The listing builds one solid part. Answer for the finished solid, in the listing's coordinates (mm). Face numbers are marked on the shaded views. Give positions to 0.01 mm unless a question says otherwise; leave off trailing zeros. Loops run counter-clockwise (first coordinate to the right, second up) from the corner with the lowest first, then second, coordinate; pieces in that order, holes last. Notation, with made-up numbers: (34, -39) - (49, -39) arc R24 ccw to (49, -28) - close; hole circle Ø8 at (84.5, -18). An arc over 180 degrees is marked (long way). Answer as CSV lines item,"result". Start each with the question number.
1) For a pull along Y with two mould halves and no side action, classify the marked faces 1, 2, 3 and 4 as pulls with the +Y half, pulls with the -Y half, needs draft (parallel to the pull), parting line crosses it, or undercut.
2) Find the intervals of material crossed by line 1 along Y through (x, z) = (2.3, 18); line 2 along X through (y, z) = (4, -6.5); line 3 along X through (y, z) = (13.5, -3.5), in increasing order.
3) Flat-ended cylindrical pins translate along their axes: pin 1 (2 mm diameter, centred on y = 14.5, z = -0.5, fed in from +X); pin 2 (1.5 mm diameter, centred on x = 1.5, y = -4.5, fed in from +Z); pin 3 (3 mm diameter, centred on y = -8.5, z = -1, fed in from -X). Find the tip coordinate at first contact, or state that the pin passes through.
4) A cutting plane is placed at B-B (z = 7). Determine the outline of the cut face in (x, y).
5) A cutting plane is placed at A-A (y = 0). Determine the outline of the cut face in (x, z).
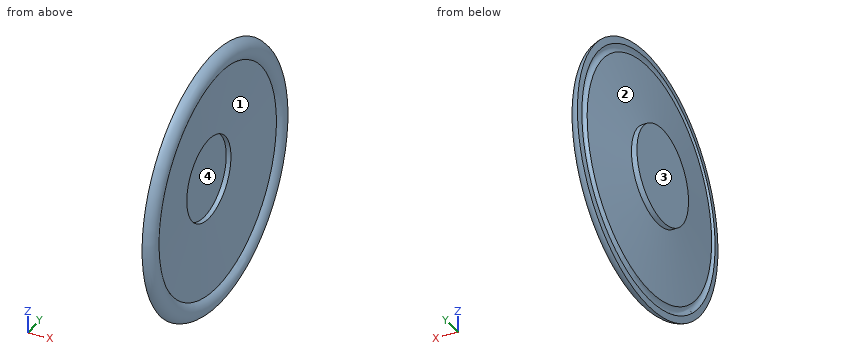
```python
from build123d import *


with BuildPart() as part:
    # Sketch1 → Revolve-Thin3 (revolve)
    with BuildSketch(Plane(origin=(0, 0, 0), x_dir=(1, 0, 0), z_dir=(0, 1, 0))):
        with BuildLine():
            Line((-0.794424497, -7), (-0.794424497, 0))
            Line((-0.794424497, 0), (0, 0))
            Line((0, 0), (1.142372775, 9.900564049))
            ThreePointArc((1.142372775, 9.900564049), (1.801141725, 10.423035974), (1.278669799, 11.081804924))
            Line((1.278669799, 11.081804924), (1.393293907, 12.07521386))
            ThreePointArc((1.393293907, 12.07521386), (2.765201716, 10.845477658), (2.061567501, 9.142750125))
            Line((2.061567501, 9.142750125), (0.891250179, -1))
            Line((0.891250179, -1), (0.205575503, -1))
            Line((0.205575503, -1), (0.205575503, -7))
            Line((0.205575503, -7), (-0.794424497, -7))
        make_face()
    revolve(axis=Axis((-0.794424497, 0, 7), (1, 0, 0)))


solid = part.part
```
Ans:
1,face 1,"undercut"
1,face 2,"parting line crosses it"
1,face 3,"needs draft"
1,face 4,"undercut"
2,line 1,"-15.07 to -12.07, 12.07 to 15.07"
2,line 2,"0.82 to 1.82"
2,line 3,"1.66 to 2.76"
3,pin 1,"x = 2.8"
3,pin 2,"z = 25.7"
3,pin 3,"x = 0.37"
4,outline,"(-0.79, -7) - (0, -7) - (1.14, -16.9) arc R0.59 cw to (1.28, -18.08) - (1.39, -19.08) arc R1.59 ccw to (2.06, -16.14) - (0.89, -6) - (0.21, -6) - (0.21, 6) - (0.89, 6) - (2.06, 16.14) arc R1.59 ccw to (1.39, 19.08) - (1.28, 18.08) arc R0.59 cw to (1.14, 16.9) - (0, 7) - (-0.79, 7) - close"
5,outline,"(-0.79, 0) - (0, 0) - (1.14, -9.9) arc R0.59 cw to (1.28, -11.08) - (1.39, -12.08) arc R1.59 ccw to (2.06, -9.14) - (0.89, 1) - (0.21, 1) - (0.21, 13) - (0.89, 13) - (2.06, 23.14) arc R1.59 ccw to (1.39, 26.08) - (1.28, 25.08) arc R0.59 cw to (1.14, 23.9) - (0, 14) - (-0.79, 14) - close"
